Here's how the part is built. I have some questions about the finished solid (model axes, mm). Face numbers are marked on the shaded views. A direction names the side the tool comes from. Round coordinates to 2 decimals unless told otherwise and drop trailing zeros. Order: outer loops, then holes, each group sorted by start corner. A loop starts at its lowest first (then second) coordinate and runs counter-clockwise, first axis right, second up. Notation, with made-up numbers: M 69,82.5 L 75,82.5 A10 ccw 75,91.5 Z; hole C 79.5,11.25 d7. An arc over 180 degrees is marked long. Write item = value, one per line. Start each with the question number.
Item 1: I'm going to push flat-ended pins straight in: P1, Ø9, axis at x = -1.5, z = -3, coming from the -Y side; P2, Ø2, axis at x = -2, z = -10.5, coming from the -Y side; P3, Ø3, axis at x = -10.5, y = -8.5, coming from the +Z side; P4, Ø3.5, axis at x = -5.5, y = -9.5, coming from the -Z side. Where does each tip first touch, or does it pass through?
Item 2: We'd pull the mould along X, two halves only. Please class the marked faces 4, 5, 6 and 7: pulls with the +X half, pulls with the -X half, needs draft (parallel to the pull), parting line crosses it, or undercut.
Item 3: I want a section at C-C, the plane z = 0. List the corners of the cut face in (x, y) for me, plus the area to 3 significant figures.
Item 4: I want a section at D-D, the plane y = -4. List the corners of the cut face in (x, z) for me.
Item 5: For the marked faces 1, 2 and 3, which set-ups out of +Z, -Z, +X, -X, +Y, -Y let a thin tool reach every point of the face, with its end or its side?
Item 6: Please list where these lines run through material, in increasing order: L1, parallel to Y at x = -10.5, z = 16.25; L2, parallel to Y at x = 5, z = 1.5; L3, parallel to Y at x = 8.5, z = -8.
Item 7: I want a section at A-A, the plane y = -8.5. List the corners of the cut face in (x, z) for me.
Item 8: I want a section at B-B, the plane x = 10.5. List the corners of the cut face in (y, z) for me.
```python
from build123d import *

# Parameters (mm, degrees)
SKETCH1_W           = 28
SKETCH1_H           = 28
SKETCH1_R           = 9
BOSS_EXTRUDE3_DEPTH = 5
BOSS_EXTRUDE4_START = 2
SKETCH1_4_W         = 28
SKETCH1_4_H         = 28
SKETCH1_4_R         = 9
SKETCH1_4_H_2       = 5
BOSS_EXTRUDE4_DEPTH = 2
SKETCH1_5_W         = 28
SKETCH1_5_H         = 5
BOSS_EXTRUDE5_DEPTH = 12
SKETCH2_R           = 2
CUT_EXTRUDE1_DEPTH  = 34.526109228
BOSS_EXTRUDE6_START = 2
SKETCH2_3_W         = 28
SKETCH2_3_H         = 7
SKETCH2_3_R         = 2
BOSS_EXTRUDE6_DEPTH = 2


with BuildPart() as part:
    # Sketch1 → Boss-Extrude3 (new body)
    with BuildSketch(Plane(origin=(0, 0, 0), x_dir=(1, 0, 0), z_dir=(0, 1, 0))):
        Rectangle(SKETCH1_W, SKETCH1_H)
        with Locations(Location((0, 0, 0), (0, 0, 270))):
            Circle(SKETCH1_R, mode=Mode.SUBTRACT)
    extrude(amount=-BOSS_EXTRUDE3_DEPTH)

    # Sketch1_4 → Boss-Extrude4 (add)
    # profile 1 of 3: a face of its own
    with BuildSketch(Plane(origin=(0, 0, 0), x_dir=(1, 0, 0), z_dir=(0, 1, 0)).offset(BOSS_EXTRUDE4_START)):
        Rectangle(SKETCH1_4_W, SKETCH1_4_H)
        with Locations(Location((0, 0, 0), (0, 0, 270))):
            Circle(SKETCH1_4_R, mode=Mode.SUBTRACT)
    # profile 2 of 3: a face of its own
    with BuildSketch(Plane(origin=(0, 0, 0), x_dir=(1, 0, 0), z_dir=(0, 1, 0)).offset(BOSS_EXTRUDE4_START)):
        with Locations((0, -16.5)):
            Rectangle(SKETCH1_4_W, SKETCH1_4_H_2)
    # profile 3 of 3: a face of its own
    with BuildSketch(Plane(origin=(0, 0, 0), x_dir=(1, 0, 0), z_dir=(0, 1, 0)).offset(BOSS_EXTRUDE4_START)):
        with Locations(Location((0, 0, 0), (0, 0, 270))):
            Circle(SKETCH1_4_R)
    extrude(amount=-BOSS_EXTRUDE4_DEPTH)

    # Sketch1_5 → Boss-Extrude5 (add)
    with BuildSketch(Plane(origin=(0, 0, 0), x_dir=(1, 0, 0), z_dir=(0, 1, 0))):
        with Locations((0, -16.5)):
            Rectangle(SKETCH1_5_W, SKETCH1_5_H)
    extrude(amount=-BOSS_EXTRUDE5_DEPTH)

    # Sketch2 → Cut-Extrude1 (cut, through all)
    with BuildSketch(Plane(origin=(0, 0, 14), x_dir=(-1, 0, 0), z_dir=(0, 0, -1))):
        with Locations((-10.5, -8.5)):
            Circle(SKETCH2_R)
        with Locations((10.5, -8.5)):
            Circle(SKETCH2_R)
    extrude(amount=-CUT_EXTRUDE1_DEPTH, mode=Mode.SUBTRACT)

    # Sketch2_3 → Boss-Extrude6 (add)
    with BuildSketch(Plane(origin=(0, 0, 14), x_dir=(-1, 0, 0), z_dir=(0, 0, -1)).offset(BOSS_EXTRUDE6_START)):
        with Locations((0, -8.5)):
            Rectangle(SKETCH2_3_W, SKETCH2_3_H)
        with Locations((-10.5, -8.5)):
            Circle(SKETCH2_3_R, mode=Mode.SUBTRACT)
        with Locations((10.5, -8.5)):
            Circle(SKETCH2_3_R, mode=Mode.SUBTRACT)
    extrude(amount=-BOSS_EXTRUDE6_DEPTH)


solid = part.part
```
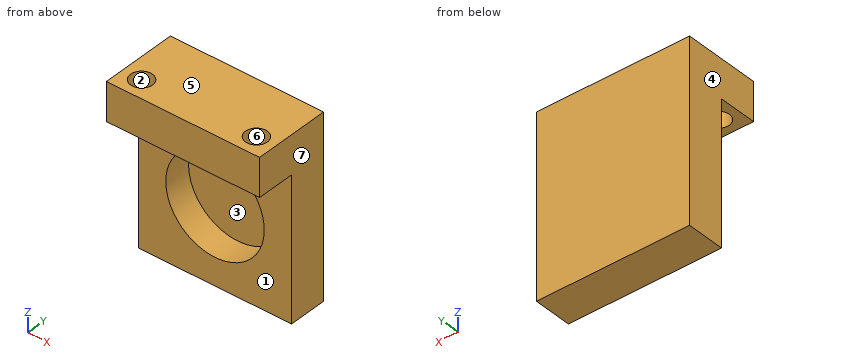
Filled in:
q1.P1 = 0
q1.P2 = -5
q1.P3 = through
q1.P4 = 12
q2.face_4 = pulls with the -X half
q2.face_5 = needs draft
q2.face_6 = undercut
q2.face_7 = pulls with the +X half
q3.outline = M -14,-5 L -9,-5 L -9,0 L 9,0 L 9,-5 L 14,-5 L 14,2 L -14,2 Z
q3.area = 106 mm^2
q4.outline = M -14,-14 L 14,-14 L 14,19 L -14,19 Z; hole C 0,0 d18
q5.face_1 = -Z, +X, -X, -Y
q5.face_2 = +Z, -Z
q5.face_3 = -Y
q6.L1 = -12 to -10.5, -6.5 to 2
q6.L2 = 0 to 2
q6.L3 = -5 to 2
q7.outline = M -14,12 L -12.5,12 L -12.5,19 L -14,19 Z; M -8.5,12 L 8.5,12 L 8.5,19 L -8.5,19 Z; M 12.5,12 L 14,12 L 14,19 L 12.5,19 Z
q8.outline = M -12,12 L -10.5,12 L -10.5,19 L -12,19 Z; M -6.5,12 L -5,12 L -5,-14 L 2,-14 L 2,19 L -6.5,19 Z
